```python
from build123d import *

# Parameters (mm, degrees)
SKETCH1_W           = 15
SKETCH1_H           = 15
BOSS_EXTRUDE1_DEPTH = 4
SKETCH3_R           = 1
CUT_EXTRUDE1_DEPTH  = 22.587033145
SKETCH4_R           = 4.5
CUT_EXTRUDE2_DEPTH  = 22.587033145
FILLET1_R           = 3


with BuildPart() as part:
    # Sketch1 → Boss-Extrude1 (new body)
    with BuildSketch(Plane(origin=(0, 0, 0), x_dir=(1, 0, 0), z_dir=(0, 1, 0))):
        with Locations((7.5, -7.5)):
            Rectangle(SKETCH1_W, SKETCH1_H)
    extrude(amount=BOSS_EXTRUDE1_DEPTH)

    # Sketch2 → Cut-Revolve1 (revolve, cut)
    with BuildSketch(Plane(origin=(0, 4, 0), x_dir=(1, 0, 0), z_dir=(0, 1, 0))):
        with BuildLine():
            Line((12.7, -7.5), (2.3, -7.5))
            ThreePointArc((2.3, -7.5), (7.5, -12.7), (12.7, -7.5))
        make_face()
    revolve(axis=Axis((12.7, 4, 7.5), (-1, 0, 0)), mode=Mode.SUBTRACT)

    # Sketch3 → Cut-Extrude1 (cut, through all)
    with BuildSketch(Plane(origin=(0, 4, 0), x_dir=(1, 0, 0), z_dir=(0, 1, 0))):
        with Locations(Location((2.5, -12.5, 0), (0, 0, 270))):
            Circle(SKETCH3_R)
        with Locations(Location((12.5, -12.5, 0), (0, 0, 270))):
            Circle(SKETCH3_R)
        with Locations(Location((12.5, -2.5, 0), (0, 0, 270))):
            Circle(SKETCH3_R)
        with Locations(Location((2.5, -2.5, 0), (0, 0, 270))):
            Circle(SKETCH3_R)
    extrude(amount=-CUT_EXTRUDE1_DEPTH, mode=Mode.SUBTRACT)

    # Sketch4 → Cut-Extrude2 (cut, through all)
    with BuildSketch(Plane(origin=(0, 0, 0), x_dir=(-1, 0, 0), z_dir=(0, -1, 0))):
        with Locations(Location((-7.5, -7.5, 0), (0, 0, 90))):
            Circle(SKETCH4_R)
    extrude(amount=-CUT_EXTRUDE2_DEPTH, mode=Mode.SUBTRACT)

    # Fillet1
    fillet1_edges = [part.edges().sort_by_distance(p)[0] for p in [
        (0, 2, 0),
        (15, 2, 0),
        (15, 2, 15),
        (0, 2, 15),
    ]]
    fillet(fillet1_edges, radius=FILLET1_R)


solid = part.part
```
CAD build for the part. Positions are in the model's coordinates, mm. Coordinates: 2 decimals unless noted, no trailing zeros. Write each loop counter-clockwise with the first axis right and the second up, starting at its lowest first coordinate (ties: lowest second). Pieces come first, ordered by that corner, then holes.
(1) Two-plate mould, pull along X, no slides. Class faces 1 (the face through (14.1, 2.03, 14.14)), 2 (the face through (2.5, 2, 11.5)), 3 (the face through (7, 2, 15)), 4 (the face through (0, 2, 8)): +X half, -X half, draft (parallel to the pull), parting line (faces both ways), or undercut.
(2) Drill centre lines: probe 1 along X at (y, z) = (0.5, 7.5); probe 2 along X at (y, z) = (1.9, 3.75); probe 3 along Z at (x, y) = (5.25, 0.85). Where is each one in solid material? Low to high.
(3) Cut at B-B, the plane z = 7.5. List the corners of the cut face in (x, y), and give its area (3 significant figures).
(4) Cut at D-D, the plane z = 2.5. List the corners of the cut face in (x, y), and give its area (3 significant figures).
(5) Cut at A-A, the plane y = 0.9. List the corners of the cut face in (x, z), and give its area (3 significant figures).
(6) Cut at C-C, the plane x = 2.5. List the corners of the cut face in (y, z).
Geometry says:
1. face 1: +X half
1. face 2: undercut
1. face 3: draft
1. face 4: -X half
2. probe 1: x = 0 to 3, 12 to 15
2. probe 2: x = 0 to 4.57, 10.43 to 15
2. probe 3: z = 0 to 3.6, 11.4 to 15
3. outline: (0, 0) - (3, 0) - (3, 1.39) arc R5.2 cw to (2.3, 4) - (0, 4) - close; (12, 0) - (15, 0) - (15, 4) - (12.7, 4) arc R5.2 cw to (12, 1.39) - close
3. area: 21.5 mm2
4. outline: (0.04, 0) - (1.5, 0) - (1.5, 4) - (0.04, 4) - close; (3.5, 0) - (11.5, 0) - (11.5, 4) - (8.93, 4) arc R1.43 cw to (6.07, 4) - (3.5, 4) - close; (13.5, 0) - (14.96, 0) - (14.96, 4) - (13.5, 4) - close
4. area: 40.5 mm2
5. outline: (0, 3) arc R3 ccw to (3, 0) - (12, 0) arc R3 ccw to (15, 3) - (15, 12) arc R3 ccw to (12, 15) - (3, 15) arc R3 ccw to (0, 12) - close; hole circle Ø2 at (2.5, 2.5); hole circle Ø2 at (2.5, 12.5); hole circle Ø9 at (7.5, 7.5); hole circle Ø2 at (12.5, 2.5); hole circle Ø2 at (12.5, 12.5)
5. area: 141 mm2
6. outline: (0, 0.04) - (4, 0.04) - (4, 1.5) - (0, 1.5) - close; (0, 3.5) - (4, 3.5) - (4, 6.07) arc R1.43 cw to (4, 8.93) - (4, 11.5) - (0, 11.5) - close; (0, 13.5) - (4, 13.5) - (4, 14.96) - (0, 14.96) - close
